CAD build for the part. Positions are in the model's coordinates, mm. Round coordinates to 2 decimals unless told otherwise and drop trailing zeros. Write each loop counter-clockwise with the first axis right and the second up, starting at its lowest first coordinate (ties: lowest second). Pieces come first, ordered by that corner, then holes. Notation, with made-up numbers: M 48.5,62.25 L 52.5,62.25 A26 cw 52.5,94.25 Z; hole C 23,-16 d1. An arc over 180 degrees is marked long. Write each question's results on one line, items separated by ' | '. Start each with the question number.
```python
from build123d import *

# Parameters (mm, degrees)
F0_R     = 1.5
F1_DEPTH = 1
F2_R     = 5.08


with BuildPart() as f1:
    # F0 (on Top) → F1 (new body)
    with BuildSketch(Plane.XY):
        Polygon((-6.35, 12.7), (6.35, 12.7), (6.35, 16.51), (6.35, 20.32), (-6.35, 20.32), align=None)
        with Locations((0, 16.51)):
            Circle(F0_R, mode=Mode.SUBTRACT)
        Polygon((31.75, -12.7), (31.75, 12.7), (6.35, 12.7), (-6.35, 12.7), (-31.75, 12.7), (-31.75, -12.7), (-6.35, -12.7), (6.35, -12.7), align=None)
        Polygon((6.35, -16.51), (6.35, -12.7), (-6.35, -12.7), (-6.35, -20.32), (6.35, -20.32), align=None)
        with Locations((0, -16.51)):
            Circle(F0_R, mode=Mode.SUBTRACT)
    extrude(amount=F1_DEPTH)

    # F2
    f2_edges = [f1.edges().sort_by_distance(p)[0] for p in [
        (6.35, 20.32, 0.5),
        (-6.35, 20.32, 0.5),
        (-6.35, -20.32, 0.5),
        (6.35, -20.32, 0.5),
    ]]
    fillet(f2_edges, radius=F2_R)


solid = f1.part
```
1) Saw through at B-B, the plane z = 0.15. Write the cut outline in (x, y), plus the area to 3 significant figures.
2) Saw through at A-A, the plane x = 0. Write the cut outline in (y, z), plus the area to 3 significant figures.
3) Saw through at C-C, the plane y = 16.51. Write the cut outline in (x, z), plus the area to 3 significant figures.
4) Wall check: line 1 along Y through (x, z) = (0, 0.75); line 2 along X through (y, z) = (-14.5, 0.2). Give the ranges that are in metal, low to high. Write a range as from..to.
5) Pull direction X, two halves, no side cores. Call faces 1 (the face through (0, 0, 1)), 2 (the face through (-0.195, -15.023, 0.493)), 3 (the face through (-4.901, 18.792, 0.507)): pulls with the +X half, pulls with the -X half, needs draft (parallel to the pull), parting line crosses it, or undercut.
6) Drop flat-ended pins along their axis: pin 1 Ø2.5 at (x, y) = (0, -16.51) entering from -Z; pin 2 Ø0.5 at (x, z) = (16, 0.5) entering from +Y. Give the stop position or say it passes through.
7) Saw through at D-D, the plane x = -14.5. Write the cut outline in (y, z).
Filled sheet:
1) outline: M -31.75,-12.7 L -6.35,-12.7 L -6.35,-15.24 A5.08 ccw -1.27,-20.32 L 1.27,-20.32 A5.08 ccw 6.35,-15.24 L 6.35,-12.7 L 31.75,-12.7 L 31.75,12.7 L 6.35,12.7 L 6.35,15.24 A5.08 ccw 1.27,20.32 L -1.27,20.32 A5.08 ccw -6.35,15.24 L -6.35,12.7 L -31.75,12.7 Z; hole C 0,-16.51 d3; hole C 0,16.51 d3 | area: 1,770 mm^2
2) outline: M -20.32,0 L -18.01,0 L -18.01,1 L -20.32,1 Z; M -15.01,0 L 15.01,0 L 15.01,1 L -15.01,1 Z; M 18.01,0 L 20.32,0 L 20.32,1 L 18.01,1 Z | area: 34.6 mm^2
3) outline: M -6.19,0 L -1.5,0 L -1.5,1 L -6.19,1 Z; M 1.5,0 L 6.19,0 L 6.19,1 L 1.5,1 Z | area: 9.38 mm^2
4) line 1: y = -20.32..-18.01, -15.01..15.01, 18.01..20.32 | line 2: x = -6.35..6.35
5) face 1: needs draft | face 2: undercut | face 3: pulls with the -X half
6) pin 1: passes through | pin 2: stops at y = 12.7
7) outline: M -12.7,0 L 12.7,0 L 12.7,1 L -12.7,1 Z
